Could you check a few things on this model? Use its own coordinates, in mm. A direction names the side the tool comes from. Coordinates: 2 decimals unless noted, no trailing zeros. Write each loop counter-clockwise with the first axis right and the second up, starting at its lowest first coordinate (ties: lowest second). Pieces come first, ordered by that corner, then holes.
```python
from build123d import *

# Parameters (mm, degrees)
BOSS_EXTRUDE1_DEPTH = 5
BOSS_EXTRUDE2_DEPTH = 25
BOSS_EXTRUDE4_DEPTH = 25
CUT_EXTRUDE1_DEPTH  = 3


with BuildPart() as part:
    # layout → Boss-Extrude1 (new body)
    with BuildSketch(Plane(origin=(0, 0, 0), x_dir=(1, 0, 0), z_dir=(0, 1, 0))):
        Polygon((0, -60), (51.961524227, -30), (51.961524227, 30), (0, 60), (-51.961524227, 30), (-51.961524227, -30), align=None)
    extrude(amount=BOSS_EXTRUDE1_DEPTH)

    # Sketch2 → Boss-Extrude2 (add)
    with BuildSketch(Plane(origin=(0, 5, 0), x_dir=(1, 0, 0), z_dir=(0, 1, 0))):
        Polygon((-51.961524227, -30), (0, -60), (51.961524227, -30), (51.961524227, 30), (0, 60), (-51.961524227, 30), align=None)
        Polygon((-46.961524227, -27.113248654), (0, -54.226497308), (46.961524227, -27.113248654), (46.961524227, 27.113248654), (0, 54.226497308), (-46.961524227, 27.113248654), align=None, mode=Mode.SUBTRACT)
    extrude(amount=BOSS_EXTRUDE2_DEPTH)

    # Sketch3 → Boss-Extrude4 (add)
    with BuildSketch(Plane(origin=(0, 5, 0), x_dir=(1, 0, 0), z_dir=(0, 1, 0))):
        Polygon((-44.461524227, 25.669872981), (-44.461524227, -25.669872981), (0, -51.339745962), (44.461524227, -25.669872981), (44.461524227, 25.669872981), (0, 51.339745962), align=None)
        Polygon((0, 47.875644347), (-41.461524227, 23.937822174), (-41.461524227, -23.937822174), (0, -47.875644347), (41.461524227, -23.937822174), (41.461524227, 23.937822174), align=None, mode=Mode.SUBTRACT)
    extrude(amount=BOSS_EXTRUDE4_DEPTH)

    # Sketch4 → Cut-Extrude1 (cut)
    with BuildSketch(Plane.ZY.offset(-41.461524227)):
        Polygon((-5, 5), (5, 5), (0, 10), align=None)
    extrude(amount=-CUT_EXTRUDE1_DEPTH, mode=Mode.SUBTRACT)


solid = part.part
```
1. If we mould it in two halves opening along X, with no side actions, what happens to faces 1 (the face through (-1, 0, -1)), 2 (the face through (51.962, 15, 0)), 3 (the face through (21.92, 17.325, 38.684))? For each: pulls with the +X half, pulls with the -X half, needs draft (parallel to the pull), parting line crosses it, or undercut.
Verdict:
face 1: needs draft
face 2: pulls with the +X half
face 3: undercut
2. I want a section at C-C on z = -15. Please give me the cut outline in (x, y).
Verdict:
outline: (-51.96, 0) - (51.96, 0) - (51.96, 30) - (46.96, 30) - (46.96, 5) - (44.46, 5) - (44.46, 30) - (41.46, 30) - (41.46, 5) - (-41.46, 5) - (-41.46, 30) - (-44.46, 30) - (-44.46, 5) - (-46.96, 5) - (-46.96, 30) - (-51.96, 30) - close
3. On a 3-axis mill with a long thin cutter (end or side, diameter ignored), from which of +Z, -Z, +X, -X, +Y, -Y can I reach the whole of each face in a straight line? I mean faces 4 (the face through (43, 8, -2)), 5 (the face through (-44.462, 17, 0)), 6 (the face through (19, 30, 44)). Say none if no direction works.
Verdict:
face 4: none
face 5: +Y
face 6: +Z, -Z, +X, -X, +Y
4. I want a section at A-A on y = 8.25. Please give me the cut outline in (x, z), plus the area to 3 significant figures.
Verdict:
outline: (-51.96, -30) - (0, -60) - (51.96, -30) - (51.96, 30) - (0, 60) - (-51.96, 30) - close; (-44.46, -25.67) - (0, -51.34) - (44.46, -25.67) - (44.46, -1.75) - (41.46, -1.75) - (41.46, -23.94) - (0, -47.88) - (-41.46, -23.94) - (-41.46, 23.94) - (0, 47.88) - (41.46, 23.94) - (41.46, 1.75) - (44.46, 1.75) - (44.46, 25.67) - (0, 51.34) - (-44.46, 25.67) - close; hole (-46.96, -27.11) - (0, -54.23) - (46.96, -27.11) - (46.96, 27.11) - (0, 54.23) - (-46.96, 27.11) - close
area: 2,600 mm2
5. I want a section at B-B on y = 27.75. Please give me the cut outline in (x, z).
Verdict:
outline: (-51.96, -30) - (0, -60) - (51.96, -30) - (51.96, 30) - (0, 60) - (-51.96, 30) - close; (-44.46, -25.67) - (0, -51.34) - (44.46, -25.67) - (44.46, 25.67) - (0, 51.34) - (-44.46, 25.67) - close; hole (-46.96, -27.11) - (0, -54.23) - (46.96, -27.11) - (46.96, 27.11) - (0, 54.23) - (-46.96, 27.11) - close; hole (-41.46, -23.94) - (0, -47.88) - (41.46, -23.94) - (41.46, 23.94) - (0, 47.88) - (-41.46, 23.94) - close
6. I want a section at D-D on x = -18. Please give me the cut outline in (y, z).
Verdict:
outline: (0, -49.61) - (30, -49.61) - (30, -43.83) - (5, -43.83) - (5, -40.95) - (30, -40.95) - (30, -37.48) - (5, -37.48) - (5, 37.48) - (30, 37.48) - (30, 40.95) - (5, 40.95) - (5, 43.83) - (30, 43.83) - (30, 49.61) - (0, 49.61) - close
7. Please list where these lines run through material, in increasing order: line 1 along X through (y, z) = (5.25, -22.5); line 2 along Z through (x, y) = (-18.5, 6.5); line 3 along X through (y, z) = (18.25, 29).
Verdict:
line 1: x = -51.96 to -46.96, -44.46 to -41.46, 41.46 to 44.46, 46.96 to 51.96
line 2: z = -49.32 to -43.55, -40.66 to -37.19, 37.19 to 40.66, 43.55 to 49.32
line 3: x = -51.96 to -43.69, -38.69 to -32.69, 32.69 to 38.69, 43.69 to 51.96
8. For pin 1 (8 mm diameter, centred on x = -7, y = 20.5, fed in from +Z); pin 2 (6 mm diameter, centred on x = -8, y = 15, fed in from +Z); pin 3 (6 mm diameter, centred on x = -18, y = 5.5, fed in from -Z), each with a flat end and sliding along its axis, tell me the tip position at first contact or that it passes through.
Verdict:
pin 1: stops at z = 58.27
pin 2: stops at z = 57.11
pin 3: stops at z = -51.34
